from build123d import *

# Parameters (mm, degrees)
SKETCH1_W           = 130
SKETCH1_H           = 130
BOSS_EXTRUDE1_DEPTH = 15
FILLET1_R           = 15
BOSS_EXTRUDE3_DEPTH = 20
BOSS_EXTRUDE4_DEPTH = 23
CUT_EXTRUDE1_DEPTH  = 50
CUT_EXTRUDE2_DEPTH  = 50
SKETCH10_R          = 3
CUT_EXTRUDE3_DEPTH  = 10


with BuildPart() as part:
    # Sketch1 → Boss-Extrude1 (new body)
    with BuildSketch(Plane.XY):
        Rectangle(SKETCH1_W, SKETCH1_H)
    extrude(amount=BOSS_EXTRUDE1_DEPTH)

    # Fillet1
    fillet1_edges = [part.edges().sort_by_distance(p)[0] for p in [
        (65, -65, 7.5),
        (-65, -65, 7.5),
        (-65, 65, 7.5),
        (65, 65, 7.5),
    ]]
    fillet(fillet1_edges, radius=FILLET1_R)

    # Sketch5 → Boss-Extrude3 (add)
    with BuildSketch(Plane.XY.offset(15)):
        Polygon((-65, 65), (65, -65), (70.504249196, -59.495750804), (-59.495750804, 70.504249196), align=None)
    extrude(amount=BOSS_EXTRUDE3_DEPTH)

    # Sketch6 → Cut-Revolve2 (revolve, cut)
    with BuildSketch(Plane(origin=(0, 0, 0), x_dir=(0, 0, 1), z_dir=(-0.707106781, -0.707106781, 0))):
        with BuildLine():
            Line((15, 91.923881554), (15, 99.514365428))
            Line((15, 99.514365428), (45.882557295, 99.514365428))
            Line((45.882557295, 99.514365428), (45.882557295, 91.923881554))
            Line((45.882557295, 91.923881554), (45.882557295, 0))
            Line((45.882557295, 0), (6.998120304, 0))
            ThreePointArc((6.998120304, 0), (9.00236559, 46.135750993), (15, 91.923881554))
        make_face()
    revolve(axis=Axis((0, 0, 45.882557295), (0, 0, 1)), mode=Mode.SUBTRACT)

    # Sketch7 → Boss-Extrude4 (add)
    with BuildSketch(Plane(origin=(0, 0, 0), x_dir=(-1, 0, 0), z_dir=(0, 0, -1))):
        Polygon((-22, -65), (22, -65), (22, -22), (65, -22), (65, 22), (22, 22), (22, 65), (-22, 65), (-22, 22), (-65, 22), (-65, -22), (-22, -22), align=None)
    extrude(amount=BOSS_EXTRUDE4_DEPTH)

    # Sketch8 → Cut-Extrude1 (cut)
    with BuildSketch(Plane.XZ.offset(22)):
        Polygon((-65, 0), (-55.807611845, -9.192388155), (-45.807611845, -9.192388155), (-40, -23), (0, -40.620002029), (40, -23), (45.807611845, -9.192388155), (55.807611845, -9.192388155), (65, 0), (68.211957708, -1.350979723), (68.682657398, -47.498818865), (-34.338090691, -46.266881669), (-70.140917764, -27.552380355), align=None)
    extrude(amount=-CUT_EXTRUDE1_DEPTH, mode=Mode.SUBTRACT)

    # Sketch9 → Cut-Extrude2 (cut)
    with BuildSketch(Plane(origin=(22, 0, 0), x_dir=(0, 0, -1), z_dir=(1, 0, 0))):
        Polygon((0, 65), (9.192388155, 55.807611845), (9.192388155, 45.807611845), (23, 40), (23, 65), align=None)
    extrude(amount=-CUT_EXTRUDE2_DEPTH, mode=Mode.SUBTRACT)

    # Sketch10 → Cut-Extrude3 (cut)
    with BuildSketch(Plane.XZ.offset(65)):
        with Locations((0, -3)):
            Circle(SKETCH10_R)
    extrude(amount=-CUT_EXTRUDE3_DEPTH, mode=Mode.SUBTRACT)


solid = part.part
Could you check a few things on this model? Use its own coordinates, in mm. A direction names the side the tool comes from. Round coordinates to 2 decimals unless told otherwise and drop trailing zeros. Loops run counter-clockwise (first coordinate to the right, second up) from the corner with the lowest first, then second, coordinate; pieces in that order, holes last. Notation, with made-up numbers: (13, 42) - (20, 42) arc R10 cw to (20, 51) - close; hole circle Ø2 at (-25.5, 62.25). An arc over 180 degrees is marked (long way). Write item = value, one per line.
1) Imagine slicing it at B-B (y = 34). Please give me the cut outline in (x, z), and give its area (3 significant figures).
Computed:
outline = (-65, 0) - (-22, 0) - (-22, -23) - (22, -23) - (22, 0) - (65, 0) - (65, 12.08) arc R530.91 cw to (-65, 12.08) - close
area = 2,240 mm2
2) Imagine slicing it at C-C (z = -3). Please give me the cut outline in (x, y).
Computed:
outline = (-62, -22) - (-22, -22) - (-22, -65) - (-3, -65) - (-3, -55) - (3, -55) - (3, -65) - (22, -65) - (22, -22) - (62, -22) - (62, 22) - (22, 22) - (22, 62) - (-22, 62) - (-22, 22) - (-62, 22) - close
3) I need wall thicknesses on line 1 along Y through (x, z) = (58.5, -4); line 2 along Z through (x, y) = (0, -57.75); line 3 along Z through (x, y) = (0, -61.5). Which ranges of each line are inside material? Lowest first, please. Write a range as from..to.
Computed:
line_1 = -22..22
line_2 = -23..-6, 0..10.14
line_3 = -23..-6, 0..10.56
4) If we mould it in two halves opening along X, with no side actions, what happens to faces 5 (the flat face through (22, -43, -11)), 6 (the cylindrical face through (-0.65, -60.07, -5.93)), 7 (the flat face through (-38, -22, -9))? For each: pulls with the +X half, pulls with the -X half, needs draft (parallel to the pull), parting line crosses it, or undercut.
Computed:
face_5 = pulls with the +X half
face_6 = undercut
face_7 = needs draft
5) I'm going to push flat-ended pins straight in: P1, Ø13, axis at x = -36, y = -33, coming from the -Z side; P2, Ø1.8, axis at x = 0.5, z = -3, coming from the -Y side; P3, Ø4, axis at y = -17.5, z = -17.5, coming from the +X side. Where does each tip first touch, or does it pass through?
Computed:
P1 = 0
P2 = -55
P3 = 43.15
6) Imagine slicing it at D-D (x = -31). Please give me the cut outline in (y, z), and give its area (3 significant figures).
Computed:
outline = (-65, 0) - (-22, 0) - (-22, -23) - (22, -23) - (22, 0) - (65, 0) - (65, 11.89) arc R531.1 cw to (-65, 11.89) - close
area = 2,210 mm2
7) On a 3-axis mill with a long thin cutter (end or side, diameter ignored), from which of +Z, -Z, +X, -X, +Y, -Y can I reach the whole of each face in a straight line? I mean faces 1 (the flat face through (51, 0, -9.192)), 2 (the flat face through (39, -22, -9)), 3 (the flat face through (-22, -44, -11)), 4 (the flat face through (-44, 44, 0)). Say none if no direction works.
Computed:
face_1 = -Z, +X, +Y, -Y
face_2 = -Z, +X, -Y
face_3 = -Z, -X, -Y
face_4 = -Z, -X, +Y
